from build123d import *

# Parameters (mm, degrees)
EXTRUDE_1_DEPTH     = 70
SKETCH_3_R          = 2.5
SKETCH_3_R_2        = 2
CUT_EXTRUDE_1_DEPTH = 82.853527719


with BuildPart() as part:
    # 草图2 → 凸台-拉伸1 (new, symmetric)
    with BuildSketch(Plane(origin=(0, 0, 0), x_dir=(1, 0, 0), z_dir=(0, 1, 0))):
        with BuildLine():
            Line((4, 0), (26, 0))
            ThreePointArc((26, 0), (28.828427125, 1.171572875), (30, 4))
            Line((30, 4), (30, 26))
            ThreePointArc((30, 26), (28.828427125, 28.828427125), (26, 30))
            Line((26, 30), (4, 30))
            ThreePointArc((4, 30), (1.171572875, 28.828427125), (0, 26))
            Line((0, 26), (0, 4))
            ThreePointArc((0, 4), (1.171572875, 1.171572875), (4, 0))
        make_face()
        with BuildLine():
            Line((4, 2), (26, 2))
            ThreePointArc((26, 2), (27.414213562, 2.585786438), (28, 4))
            Line((28, 4), (28, 26))
            ThreePointArc((28, 26), (27.414213562, 27.414213562), (26, 28))
            Line((26, 28), (4, 28))
            ThreePointArc((4, 28), (2.585786438, 27.414213562), (2, 26))
            Line((2, 26), (2, 4))
            ThreePointArc((2, 4), (2.585786438, 2.585786438), (4, 2))
        make_face(mode=Mode.SUBTRACT)
    extrude(amount=EXTRUDE_1_DEPTH, both=True)

    # 草图3 → 切除-拉伸1 (cut, through all)
    with BuildSketch(Plane.XY):
        with Locations((10, 9.5)):
            Circle(SKETCH_3_R)
        with Locations((20, 9.5)):
            Circle(SKETCH_3_R_2)
        with Locations((20, -15.5)):
            Circle(SKETCH_3_R_2)
        with Locations((20, -62.5)):
            Circle(SKETCH_3_R_2)
    extrude(amount=-CUT_EXTRUDE_1_DEPTH, mode=Mode.SUBTRACT)


solid = part.part
Work out the finished part from the listing and answer in its coordinate system (mm). A direction names the side the tool comes from. Coordinates: 2 decimals unless noted, no trailing zeros. Loops run counter-clockwise (first coordinate to the right, second up) from the corner with the lowest first, then second, coordinate; pieces in that order, holes last. Notation, with made-up numbers: M 77.25,40 L 120.25,40 A29 ccw 120.25,63 Z; hole C 20,-1.5 d11. An arc over 180 degrees is marked long. Answer in a Markdown table with one row per item. Add a question column.
1. Find section C-C, the plane x = 10. Write down the section's boundary in (y, z), then the cut area to 3 significant figures.
2. The mould has two halves that part along Y. Classify faces 1 (the flat face through (1, 70, -15)), 2 (the flat face through (15, 1, -2)), 3 (the cylindrical face through (19.74, -60.517, -28.986)): pulls with the +Y half, pulls with the -Y half, needs draft (parallel to the pull), parting line crosses it, or undercut.
3. A tool of negligible diameter and unlimited length cuts with its end or side. For faces 4 (the cylindrical face through (18.526, 10.852, -0.986)), 5 (the flat face through (15, 1, -28)), from which of +Z, -Z, +X, -X, +Y, -Y can it reach the whole face along a straight path? Write none if from no direction.
4. Find section B-B, the plane y = -62.5. Write down the section's boundary in (x, z), then the cut area to 3 significant figures.
5. A flat-ended cylindrical pin translates along its axis: P1, Ø3, axis at x = 20, y = -62.5, coming from the +Z side. Find the tip coordinate at first contact, or state that the pin passes through.
6. Find section A-A, the plane z = -23.5. Write down the section's boundary in (x, y), then the cut area to 3 significant figures.
7. Find section D-D, the plane x = 23.25. Write down the section's boundary in (y, z), then the cut area to 3 significant figures.
8. Consider L1, parallel to Y at x = 20, z = -1.05; L2, parallel to X at y = 27, z = -13.75; L3, parallel to Z at x = 4.25, y = -59.5. Determine where each line is inside the solid, lowest interval first.
Reported:
| question | item | result |
|---|---|---|
| 1 | outline | M -70,-30 L 7,-30 L 7,-28 L -70,-28 Z; M -70,-2 L 7,-2 L 7,0 L -70,0 Z; M 12,-30 L 70,-30 L 70,-28 L 12,-28 Z; M 12,-2 L 70,-2 L 70,0 L 12,0 Z |
| 1 | area | 540 mm^2 |
| 2 | face 1 | pulls with the +Y half |
| 2 | face 2 | needs draft |
| 2 | face 3 | undercut |
| 3 | face 4 | +Z, -Z |
| 3 | face 5 | +Y, -Y |
| 4 | outline | M 0,-26 A4 ccw 4,-30 L 18,-30 L 18,-28 L 4,-28 A2 cw 2,-26 L 2,-4 A2 cw 4,-2 L 18,-2 L 18,0 L 4,0 A4 ccw 0,-4 Z; M 22,-30 L 26,-30 A4 ccw 30,-26 L 30,-4 A4 ccw 26,0 L 22,0 L 22,-2 L 26,-2 A2 cw 28,-4 L 28,-26 A2 cw 26,-28 L 22,-28 Z |
| 4 | area | 198 mm^2 |
| 5 | P1 | passes through |
| 6 | outline | M 0,-70 L 2,-70 L 2,70 L 0,70 Z; M 28,-70 L 30,-70 L 30,70 L 28,70 Z |
| 6 | area | 560 mm^2 |
| 7 | outline | M -70,-30 L 70,-30 L 70,-28 L -70,-28 Z; M -70,-2 L 70,-2 L 70,0 L -70,0 Z |
| 7 | area | 560 mm^2 |
| 8 | L1 | y = -70 to -64.5, -60.5 to -17.5, -13.5 to 7.5, 11.5 to 70 |
| 8 | L2 | x = 0 to 2, 28 to 30 |
| 8 | L3 | z = -30 to -28, -2 to 0 |
